from build123d import *

# Parameters (mm, degrees)
EXTRUDE_1_DEPTH     = 3
SKETCH_2_R          = 2.15
SKETCH_2_R_2        = 1.65
CUT_EXTRUDE_1_DEPTH = 3
FILLET_1_R          = 5


with BuildPart() as part:
    # 草图1 → 凸台-拉伸1 (new body)
    with BuildSketch(Plane.XY):
        Polygon((0, 0), (0, 154.3), (50, 104.3), (50, 0), align=None)
    extrude(amount=EXTRUDE_1_DEPTH)

    # 草图2 → 切除-拉伸1 (cut)
    with BuildSketch(Plane.XY.offset(3)):
        with Locations((8.5, 10)):
            Circle(SKETCH_2_R)
        with Locations((41.5, 10)):
            Circle(SKETCH_2_R)
        with Locations((8.5, 131.657864376)):
            Circle(SKETCH_2_R)
        with Locations((8.5, 100.45)):
            Circle(SKETCH_2_R_2)
        with Locations((8.5, 70.95)):
            Circle(SKETCH_2_R_2)
        with Locations((41.5, 70.95)):
            Circle(SKETCH_2_R_2)
        with Locations((41.5, 100.45)):
            Circle(SKETCH_2_R_2)
    extrude(amount=-CUT_EXTRUDE_1_DEPTH, mode=Mode.SUBTRACT)

    # 圆角1
    fillet_1_edges = [part.edges().sort_by_distance(p)[0] for p in [
        (0, 154.3, 1.5),
    ]]
    fillet(fillet_1_edges, radius=FILLET_1_R)


solid = part.part
Read the model definition and answer for the solid it produces. Units are mm, in the model's axes. Round coordinates to 2 decimals unless told otherwise and drop trailing zeros. Loops run counter-clockwise (first coordinate to the right, second up) from the corner with the lowest first, then second, coordinate; pieces in that order, holes last. Notation, with made-up numbers: (56.5, 41.25) - (84.5, 41.25) arc R13 ccw to (84.5, 49.25) - close; hole circle Ø7 at (75.25, -4). An arc over 180 degrees is marked (long way). One line per question, with ' | ' between items. Start each with the question number.
Q1. For a pull along Y with two mould halves and no side action, classify faces 1 (the cylindrical face through (8.285, 72.586, 1.521)), 2 (the flat face through (25, 58, 0)), 3 (the flat face through (29, 125.3, 1.5)) as +Y half, -Y half, draft (parallel to the pull), parting line (faces both ways), or undercut.
Q2. Section D-D on y = 70.95 is taken. Give the vertices of the cut face in (x, z).
Q3. Find the intervals of material crossed by L1, parallel to X at y = 70.95, z = 0.7; L2, parallel to Y at x = 8.5, z = 1.25; L3, parallel to X at y = 99, z = 1.35, in increasing order.
Q4. Section B-B on x = 41.5 is taken. Give the vertices of the cut face in (y, z), plus the area to 3 significant figures.
Q5. Section A-A on y = 10 is taken. Give the vertices of the cut face in (x, z).
Q6. Section C-C on z = 0.6 is taken. Give the vertices of the cut face in (x, y).
Established:
1) face 1: undercut | face 2: draft | face 3: +Y half
2) outline: (0, 0) - (6.85, 0) - (6.85, 3) - (0, 3) - close; (10.15, 0) - (39.85, 0) - (39.85, 3) - (10.15, 3) - close; (43.15, 0) - (50, 0) - (50, 3) - (43.15, 3) - close
3) L1: 0 to 6.85, 10.15 to 39.85, 43.15 to 50 | L2: 0 to 7.85, 12.15 to 69.3, 72.6 to 98.8, 102.1 to 129.51, 133.81 to 145.8 | L3: 0 to 7.71, 9.29 to 40.71, 42.29 to 50
4) outline: (0, 0) - (7.85, 0) - (7.85, 3) - (0, 3) - close; (12.15, 0) - (69.3, 0) - (69.3, 3) - (12.15, 3) - close; (72.6, 0) - (98.8, 0) - (98.8, 3) - (72.6, 3) - close; (102.1, 0) - (112.8, 0) - (112.8, 3) - (102.1, 3) - close | area: 306 mm²
5) outline: (0, 0) - (6.35, 0) - (6.35, 3) - (0, 3) - close; (10.65, 0) - (39.35, 0) - (39.35, 3) - (10.65, 3) - close; (43.65, 0) - (50, 0) - (50, 3) - (43.65, 3) - close
6) outline: (0, 0) - (50, 0) - (50, 104.3) - (8.54, 145.76) arc R5 ccw to (0, 142.23) - close; hole circle Ø4.3 at (8.5, 10); hole circle Ø4.3 at (8.5, 131.66); hole circle Ø3.3 at (8.5, 70.95); hole circle Ø3.3 at (8.5, 100.45); hole circle Ø4.3 at (41.5, 10); hole circle Ø3.3 at (41.5, 70.95); hole circle Ø3.3 at (41.5, 100.45)
